Geometry: final body of the model. Coordinates: model frame, mm. Face numbers are marked on the shaded views. A direction names the side the tool comes from. Give positions to 0.01 mm unless a question says otherwise; leave off trailing zeros. Write each loop counter-clockwise with the first axis right and the second up, starting at its lowest first coordinate (ties: lowest second). Pieces come first, ordered by that corner, then holes. Notation, with made-up numbers: (-33.75, -14.5) -> (21.25, -14.5) arc R12 ccw to (21.25, 7.5) -> close; hole circle Ø9 at (73.5, -3.75). An arc over 180 degrees is marked (long way). Answer as a JSON object with one key per item and string values. Group by question number.
(1) Contact query for flat-ended pins moving along their axis: pin 1 Ø0.6 at (y, z) = (9, 4.5) entering from +X; pin 2 Ø3 at (x, z) = (-6, 18) entering from -Y; pin 3 Ø6 at (y, z) = (2.5, 17) entering from +X; pin 4 Ø6 at (x, y) = (-13.5, 2.5) entering from -Z. Output: stop coordinate, or through.
(2) Draft query along X for the marked faces 1, 2 and 3. Return one class per face: +X half, -X half, draft (parallel to the pull), parting line (faces both ways), or undercut.
(3) Set-up query: the marked faces 4 and 5. Return all of +Z, -Z, +X, -X, +Y, -Y with unobstructed straight access to the full face (end or side cutting, diameter ignored); none if empty.
(4) Section query D-D on z = 6.25. Output: boundary loops of the cut face in (x, y).
(5) Section query A-A on z = 9.5. Output: boundary loops of the cut face in (x, y), plus the area to 3 significant figures.
(6) Section query B-B on z = 13.75. Output: boundary loops of the cut face in (x, y).
(7) Section query C-C on y = 0. State how many separate pieces and enclosed holes the cut face has, plus the area to 3 significant figures.
(8) Material intervals for probe 1 along Y at (x, z) = (0, 16.5); probe 2 along X at (y, z) = (0.25, 6.5); probe 3 along Y at (x, z) = (-4, 10.25), sorted ascending.
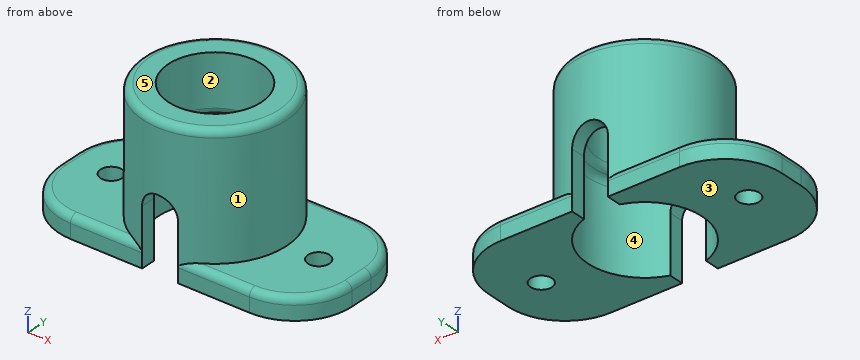
Autodesk Inventor part; units mm, degrees
ref_plane "YZ Plane" through (0, 0, 0) normal (1, 0, 0) x (0, 1, 0)
ref_plane "XZ Plane" through (0, 0, 0) normal (0, 1, 0) x (-1, 0, 0)
ref_plane "XY Plane" through (0, 0, 0) normal (0, 0, 1) x (1, 0, 0)
sketch "スケッチ1" plane through (0, 0, 0) normal (0, 0, 1) x (1, 0, 0)
  circle A0 centre (0, 0) radius 8
  circle A1 centre (0, 0) radius 10
  dimension "d0" = 16
  dimension "d1" = 2
extrude "押し出し1" add sketch "スケッチ1" along normal blind 12
sketch "スケッチ2" plane through (0, 0, 12) normal (0, 0, 1) x (1, 0, 0)
  circle A0 centre (0, 0) radius 6.5
  circle A1 centre (0, 0) radius 10
  circle A2 centre (0, 0) radius 10
  dimension "d4" = 13
extrude "押し出し2" add sketch "スケッチ2" along normal blind 8.1
sketch "スケッチ3" plane through (0, 0, 0) normal (0, 1, 0) x (-1, 0, 0)
  line L0 (10, 0) -> (-10, 0)
  line L1 (2.5, 0) -> (2.5, 8)
  arc A0 (2.5, 8) -> (-2.5, 8) centre (0, 8) ccw
  line L2 (-2.5, 8) -> (-2.5, 0)
  line L3 (2.5, 0) -> (-2.5, 0)
  line L4 (0, -2.1) -> (0, 12.6)
  point P0 (0, 0)
  dimension "d7" = 5
  dimension "d8" = 8
extrude "押し出し3" cut sketch "スケッチ3" along normal through all both and the other way through all
fillet "フィレット1" radius 1 2 edges at (-8, 0, 12) (-6.5, 0, 12)
fillet "フィレット2" radius 1 1 edges at (-10, 0, 20.1)
sketch "スケッチ4" plane through (0, 0, 0) normal (0, 0, -1) x (-1, 0, 0)
  line L0 (2.5, -9.6825) -> (2.5, -7.5993)
  line L1 (2.5, -9.6825) -> (20.5, -9.6825)
  circle A0 centre (0, 0) radius 10
  line L2 (2.5, 9.6825) -> (20.5, 9.6825)
  line L3 (20.5, 9.6825) -> (20.5, -9.6825)
  line L4 (2.5, 7.5993) -> (2.5, 9.6825)
  arc A1 (2.5, -9.6825) -> (2.5, 9.6825) centre (0, 0) ccw
  line L5 (0, -14) -> (0, 14)
  line L6 (-2.5, -9.6825) -> (-20.5, -9.6825)
  line L7 (-2.5, 9.6825) -> (-20.5, 9.6825)
  line L8 (-20.5, 9.6825) -> (-20.5, -9.6825)
  arc A2 (-2.5, 9.6825) -> (-2.5, -9.6825) centre (0, 0) ccw
  point P0 (-2.5, -9.6825)
  dimension "d13" = 18
extrude "押し出し4" add sketch "スケッチ4" against normal blind 3 contours A0 L2 L3 L1 | L6 L8 L7 A0
fillet "フィレット3" radius 8 4 edges at (20.5, 9.6825, 1.5) (20.5, -9.6825, 1.5) (-20.5, -9.6825, 1.5) (-20.5, 9.6825, 1.5)
fillet "フィレット4" radius 1 10 edges at (-18.1569, -7.3393, 3) (-7.5, -9.6825, 3) (-18.1569, 7.3393, 3) (-7.5, 9.6825, 3) (-20.5, 0, 3) (18.1569, 7.3393, 3) (7.5, 9.6825, 3) (18.1569, -7.3393, 3) (7.5, -9.6825, 3) (20.5, 0, 3)
sketch "スケッチ5" plane through (0, 0, 3) normal (0, 0, 1) x (1, 0, 0)
  circle A0 centre (14.5, 0) radius 1.5
  circle A1 centre (0, 0) radius 10
  line L0 (-28.7, 0) -> (28.7, 0)
  line L1 (0, -14.0024) -> (0, 14.0024)
  circle A2 centre (-14.5, 0) radius 1.5
  dimension "d18" = 3
  dimension "d19" = 3
extrude "押し出し5" cut sketch "スケッチ5" against normal through all contours L0 A0 | A0 L0 | A2 L0 | L0 A2
properties part number "cover.ver1"
Answer list:
{
 "1": {"pin 1": "x = 4.93", "pin 2": "y = -8.93", "pin 3": "x = 10", "pin 4": "z = 0"},
 "2": {"face 1": "parting line", "face 2": "undercut", "face 3": "draft"},
 "3": {"face 4": "-Z", "face 5": "+Z, +X, -X, +Y, -Y"},
 "4": {"outline": "(-2.5, -9.68) -> (-2.5, -7.6) arc R8 cw to (-2.5, 7.6) -> (-2.5, 9.68) arc R10 ccw to start; (2.5, -9.68) arc R10 ccw to (2.5, 9.68) -> (2.5, 7.6) arc R8 cw to (2.5, -7.6) -> close"},
 "5": {"outline": "(-2, -9.8) -> (-2, -7.75) arc R8 cw to (-2, 7.75) -> (-2, 9.8) arc R10 ccw to start; (2, -9.8) arc R10 ccw to (2, 9.8) -> (2, 7.75) arc R8 cw to (2, -7.75) -> close", "area": "97.0 mm2"},
 "6": {"outline": "circle Ø20 at (0, 0); hole circle Ø13 at (0, 0)"},
 "7": {"separate pieces": "4", "enclosed holes": "0", "area": "149 mm2"},
 "8": {"probe 1": "-10 to -6.5, 6.5 to 10", "probe 2": "-10 to -8, 8 to 10", "probe 3": "-9.17 to -6.93, 6.93 to 9.17"}
}
